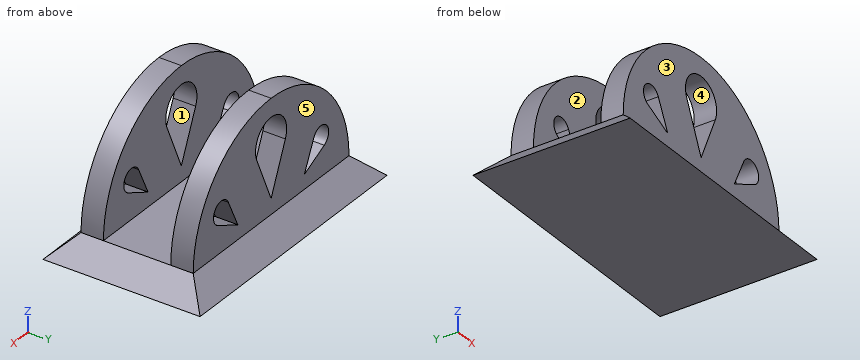
```python
from build123d import *

# Parameters (mm, degrees)
F2_W     = 100
F2_H     = 50
F0_W     = 120
F0_H     = 70
F6_DEPTH = 10


with BuildPart() as f3:
    # F2 (on offset) → F3 section 0
    with BuildSketch(Plane.XY.offset(10)):
        Rectangle(F2_W, F2_H)
    # F0 (on Top) → F3 section 1
    with BuildSketch(Plane.XY):
        Rectangle(F0_W, F0_H)
    loft()

    # F5 (on offset) → F6 (join)
    with BuildSketch(Plane.XZ.offset(-25)):
        with BuildLine():
            Line((-50, 10), (50, 10))
            ThreePointArc((50, 10), (35.355339, 45.355339), (0, 60))
            ThreePointArc((0, 60), (-35.355339, 45.355339), (-50, 10))
        make_face()
        with BuildLine():
            Line((-27.4604, 29.182527), (-21.365643, 16.421104))
            Line((-21.365643, 16.421104), (-34.127067, 22.515861))
            ThreePointArc((-34.127067, 22.515861), (-35.507778, 30.563239), (-27.4604, 29.182527))
        make_face(mode=Mode.SUBTRACT)
        with BuildLine():
            ThreePointArc((-9.165151, 37.865514), (0, 51.865514), (9.165151, 37.865514))
            Line((9.165151, 37.865514), (0, 16.865514))
            Line((0, 16.865514), (-9.165151, 37.865514))
        make_face(mode=Mode.SUBTRACT)
        with BuildLine():
            ThreePointArc((27.4604, 29.182527), (35.507778, 30.563239), (34.127067, 22.515861))
            Line((34.127067, 22.515861), (21.365643, 16.421104))
            Line((21.365643, 16.421104), (27.4604, 29.182527))
        make_face(mode=Mode.SUBTRACT)
    extrude(amount=F6_DEPTH)

    # F7: F3 across plane


with BuildPart() as f3_1:
    add(f3.part)
    add(f3.part.mirror(Plane.XZ))


solid = f3_1.part
```
Part model, mm, in its own coordinate system. Face numbers are marked on the shaded views. A direction names the side the tool comes from. Round coordinates to 2 decimals unless told otherwise and drop trailing zeros. Loops run counter-clockwise (first coordinate to the right, second up) from the corner with the lowest first, then second, coordinate; pieces in that order, holes last. Notation, with made-up numbers: (38.5, 77.5) -> (87.5, 77.5) arc R11 cw to (87.5, 94.5) -> close; hole circle Ø4 at (43, 78). An arc over 180 degrees is marked (long way). Use one line per item in the form item = value. Start each with the question number.
Item 1: Tool access for the marked faces 1, 2 and 3: list every direction of +Z, -Z, +X, -X, +Y, -Y with a clear straight run to the whole face (end or side of a thin tool).
Item 2: Drop flat-ended pins along their axis: pin 1 Ø15 at (x, z) = (-22, 45.5) entering from +Y; pin 2 Ø2 at (x, y) = (-36.5, 17.5) entering from +Z; pin 3 Ø9 at (x, y) = (-4, 4.5) entering from +Z; pin 4 Ø12 at (x, z) = (0, 41.87) entering from +Y. Give the stop position or say it passes through.
Item 3: Drill centre lines: line 1 along Y through (x, z) = (-48.5, 17); line 2 along X through (y, z) = (23, 18); line 3 along X through (y, z) = (-18, 47.5). Where is each one in solid material? Low to high.
Item 4: Band-saw the part on A-A (z = 45). List the corners of the cut face in (x, y), plus the area to 3 significant figures.
Item 5: Band-saw the part on B-B (y = 17). Give the number of separate pieces and of enclosed holes in the cut face, plus the area to 3 significant figures.
Item 6: Two-plate mould, pull along X, no slides. Class the marked faces 4 and 5: released by +X, released by -X, zero draft, split by the parting line, or undercut.
Data:
q1.face_1 = +Y, -Y
q1.face_2 = +Z, +X, -X
q1.face_3 = +Z, +X, -X, -Y
q2.pin_1 = 25
q2.pin_2 = 45.21
q2.pin_3 = 10
q2.pin_4 = through
q3.line_1 = -25 to -15, 15 to 25
q3.line_2 = -49.36 to -24.67, -22.12 to -0.5, 0.5 to 22.12, 24.67 to 49.36
q3.line_3 = -33.07 to -8.26, 8.26 to 33.07
q4.outline = (-35.71, -25) -> (-9.5, -25) -> (-9.5, -15) -> (-35.71, -15) -> close; (-35.71, 15) -> (-9.5, 15) -> (-9.5, 25) -> (-35.71, 25) -> close; (9.5, -25) -> (35.71, -25) -> (35.71, -15) -> (9.5, -15) -> close; (9.5, 15) -> (35.71, 15) -> (35.71, 25) -> (9.5, 25) -> close
q4.area = 1,050 mm^2
q5.separate_pieces = 1
q5.enclosed_holes = 3
q5.area = 4,360 mm^2
q6.face_4 = undercut
q6.face_5 = zero draft
